Geometry: final body of the model. Coordinates: model frame, mm. A direction names the side the tool comes from. Round coordinates to 2 decimals unless told otherwise and drop trailing zeros. Loops run counter-clockwise (first coordinate to the right, second up) from the corner with the lowest first, then second, coordinate; pieces in that order, holes last. Notation, with made-up numbers: (65.5, 57) - (74.5, 57) arc R14 cw to (74.5, 61) - close; hole circle Ø6 at (-17.75, 20). An arc over 180 degrees is marked (long way). Use CSV: the item, a comma, the result in double quotes.
Autodesk Inventor part; units mm, degrees
ref_plane "YZ Plane" through (0, 0, 0) normal (1, 0, 0) x (0, 1, 0)
ref_plane "XZ Plane" through (0, 0, 0) normal (0, 1, 0) x (-1, 0, 0)
ref_plane "XY Plane" through (0, 0, 0) normal (0, 0, 1) x (1, 0, 0)
sketch "Sketch1" plane through (0, 0, 0) normal (0, 0, 1) x (1, 0, 0)
  line L0 (0, 0) -> (0, 9.525)
  line L1 (0, 9.525) -> (20.6375, 9.525)
  line L2 (20.6375, 9.525) -> (20.6375, 6.35)
  line L3 (149.1107, 6.35) -> (149.1107, 4.7625)
  line L4 (149.1107, 4.7625) -> (152.4, 4.7625)
  line L5 (152.4, 4.7625) -> (152.4, 6.35)
  line L6 (152.4, 6.35) -> (158.75, 6.35)
  line L7 (158.75, 6.35) -> (158.75, 0)
  line L8 (158.75, 0) -> (0, 0)
  line L9 (149.1107, 6.35) -> (127, 6.35)
  line L10 (127, 6.35) -> (26.9875, 6.35)
  line L11 (26.9875, 6.35) -> (20.6375, 6.35)
  dimension "d0" = 9.525
  dimension "d1" = 20.6375
  dimension "d2" = 158.75
  dimension "d4" = 6.35
  dimension "d7" = 4.7625
  dimension "d8" = 3.2893
  dimension "d10" = 6.35
  dimension "d11" = 100.0125
  dimension "d12" = 6.35
revolve "Revolution1" add sketch "Sketch1" angle 360 about axis through (158.75, 0, 0) along (-1, 0, 0)
thread "Thread1"
sketch "Sketch2" plane through (0, 0, 0) normal (0, 1, 0) x (-1, 0, 0)
  circle A0 centre (-10.3188, 0) radius 4.3656
  line L0 (0, 9.525) -> (0, -9.525)
  point P0 (0, 0)
  dimension "d15" = 8.7312
  dimension "d27" = 10.3187
  dimension "d28" = 9.525
hole "Hole1" at (10.3188, 0, 0) direction (0, 1, 0) diameter 8.7313 end through all
sketch "Sketch3" plane through (0, 0, 0) normal (0, 1, 0) x (-1, 0, 0)
  circle A0 centre (-10.3188, 0) radius 4.3656
  line L0 (0, 9.525) -> (0, -9.525)
  point P0 (0, 0)
  dimension "d23" = 10.3187
  dimension "d24" = 8.7312
  dimension "d26" = 9.525
hole "Hole2" at (10.3188, 0, 0) direction (0, -1, 0) diameter 8.7313 end through all
fillet "Fillet1" radius 1.5875 1 edges at (0, -9.525, 0)
properties part number "VS-004 (VISE SCREW)" material "Steel, Alloy"
Item 1: Section C-C on x = 34.5. Return the cut outline in (y, z).
Final values:
outline,"circle Ø12.7 at (0, 0)"
Item 2: Material intervals for line 1 (X direction, y = -0.25, z = 6); line 2 (X direction, y = 4, z = 0); line 3 (X direction, y = 5, z = -1.5), sorted ascending.
Final values:
line 1,"x = 0 to 149.11, 152.4 to 158.75"
line 2,"x = 0 to 5.95, 14.68 to 158.75"
line 3,"x = 0 to 6.22, 14.42 to 149.11, 152.4 to 158.75"
Item 3: Pin query (flat end, axial travel): P1, Ø8, axis at x = 75, z = 2, coming from the +Y side; P2, Ø6, axis at x = 135.5, y = 4.5, coming from the +Z side; P3, Ø1.5, axis at x = 104, z = 1.5, coming from the -Y side. Return the tip coordinate at first contact, or that it passes through.
Final values:
P1,"stops at y = 6.35"
P2,"stops at z = 6.17"
P3,"stops at y = -6.31"
Item 4: Mould query, pull axis X, two halves, no side actions, for faces 4 (the flat face through (149.111, 1, -5)), 5 (the cylindrical face through (155.62, -1.38, -6.2)), 6 (the flat face through (20.638, 6.2, 2)). Classes: released by +X, released by -X, zero draft, split by the parting line, or undercut.
Final values:
face 4,"undercut"
face 5,"zero draft"
face 6,"released by +X"
Item 5: Reachability of faces 1 (the cylindrical face through (83.97, -1.38, 6.2)), 2 (the cylindrical face through (150.78, -3.78, -2.9)), 3 (the flat face through (0, 0, 0)) from +Z, -Z, +X, -X, +Y, -Y: full face, straight path, thin tool, end or side. Return the list, or none.
Final values:
face 1,"+X"
face 2,"none"
face 3,"+Z, -Z, -X, +Y, -Y"
